```python
from build123d import *

# Parameters (mm, degrees)
BOSS_EXTRUDE1_DEPTH = 3.175
SKETCH2_R           = 4.7625
CUT_EXTRUDE1_DEPTH  = 7.35


with BuildPart() as part:
    # Sketch1 → Boss-Extrude1 (new body, symmetric)
    with BuildSketch(Plane(origin=(0, 0, 0), x_dir=(1, 0, 0), z_dir=(0, 1, 0))):
        Polygon((-58.039, -19.304), (-58.039, -58.039), (-19.304, -58.039), (-19.304, -38.1), (19.304, -38.1), (19.304, -58.039), (58.039, -58.039), (58.039, -19.304), (38.1, -19.304), (38.1, 19.304), (58.039, 19.304), (58.039, 58.039), (19.304, 58.039), (19.304, 38.1), (-19.304, 38.1), (-19.304, 58.039), (-58.039, 58.039), (-58.039, 19.304), (-38.1, 19.304), (-38.1, -19.304), align=None)
    extrude(amount=BOSS_EXTRUDE1_DEPTH, both=True)

    # Sketch2 → Cut-Extrude1 (cut, through all)
    with BuildSketch(Plane(origin=(0, 3.175, 0), x_dir=(1, 0, 0), z_dir=(0, 1, 0))):
        with Locations((-22.86, 22.86)):
            Circle(SKETCH2_R)
        with Locations((-22.86, -22.86)):
            Circle(SKETCH2_R)
        with Locations((22.86, -22.86)):
            Circle(SKETCH2_R)
        with Locations((22.86, 22.86)):
            Circle(SKETCH2_R)
    extrude(amount=-CUT_EXTRUDE1_DEPTH, mode=Mode.SUBTRACT)


solid = part.part
```
Could you check a few things on this model? Use its own coordinates, in mm. A direction names the side the tool comes from. Round coordinates to 2 decimals unless told otherwise and drop trailing zeros. Loops run counter-clockwise (first coordinate to the right, second up) from the corner with the lowest first, then second, coordinate; pieces in that order, holes last.
Q1. On a 3-axis mill with a long thin cutter (end or side, diameter ignored), from which of +Z, -Z, +X, -X, +Y, -Y can I reach the whole of each face in a straight line? I mean faces 4 (the flat face through (19.304, 0, 48)), 5 (the flat face through (-39, 0, 58.039)), 6 (the flat face through (-38.1, 0, 0)), 7 (the flat face through (38.1, 0, 0)), 8 (the flat face through (-19.304, 0, -48)). Say none if no direction works.
Q2. Thinking about a two-plate mould opening in Z: for faces 1 (the flat face through (-19.304, 0, 48)), 2 (the flat face through (0, 0, 38.1)), 3 (the flat face through (48, 0, 19.304)), which applies, pulls with the +Z half, pulls with the -Z half, needs draft (parallel to the pull), parting line crosses it, or undercut?
Q3. I want a section at C-C (x = -45). Write out the boundary of the cut face in (y, z) (3 decimals).
Q4. I want a section at B-B (y = -1.75). Write out the boundary of the cut face in (x, z) (1 decimal).
Q5. Please list where these lines run through material, in increasing order: L1, parallel to Z at x = -22.86, y = -1.5; L2, parallel to Z at x = -38.5, y = 1.25.
Q6. For P1, Ø1.9, axis at x = -4.5, y = 1, coming from the -Z side; P2, Ø1.9, axis at y = -0.5, z = -5, coming from the -X side; P3, Ø3, axis at y = 0.5, z = -8.5, coming from the +X side, each with a flat end and sliding along its axis, tell me the tip position at first contact or that it passes through.
Q7. I want a section at A-A (x = 22.86). Write out the boundary of the cut face in (y, z) (1 decimal).
Q8. I want a section at D-D (z = 46.5). Write out the boundary of the cut face in (x, y) (3 decimals).
Answer below:
1. face 4: +Z, +Y, -Y
1. face 5: +Z, +X, -X, +Y, -Y
1. face 6: -X, +Y, -Y
1. face 7: +X, +Y, -Y
1. face 8: -Z, +Y, -Y
2. face 1: needs draft
2. face 2: pulls with the +Z half
2. face 3: undercut
3. outline: (-3.175, -58.039) - (3.175, -58.039) - (3.175, -19.304) - (-3.175, -19.304) - close; (-3.175, 19.304) - (3.175, 19.304) - (3.175, 58.039) - (-3.175, 58.039) - close
4. outline: (-58, -58) - (-19.3, -58) - (-19.3, -38.1) - (19.3, -38.1) - (19.3, -58) - (58, -58) - (58, -19.3) - (38.1, -19.3) - (38.1, 19.3) - (58, 19.3) - (58, 58) - (19.3, 58) - (19.3, 38.1) - (-19.3, 38.1) - (-19.3, 58) - (-58, 58) - (-58, 19.3) - (-38.1, 19.3) - (-38.1, -19.3) - (-58, -19.3) - close; hole circle Ø9.5 at (-22.9, -22.9); hole circle Ø9.5 at (-22.9, 22.9); hole circle Ø9.5 at (22.9, -22.9); hole circle Ø9.5 at (22.9, 22.9)
5. L1: z = -58.04 to -27.62, -18.1 to 18.1, 27.62 to 58.04
5. L2: z = -58.04 to -19.3, 19.3 to 58.04
6. P1: stops at z = -38.1
6. P2: stops at x = -38.1
6. P3: stops at x = 38.1
7. outline: (-3.2, -58) - (3.2, -58) - (3.2, -27.6) - (-3.2, -27.6) - close; (-3.2, -18.1) - (3.2, -18.1) - (3.2, 18.1) - (-3.2, 18.1) - close; (-3.2, 27.6) - (3.2, 27.6) - (3.2, 58) - (-3.2, 58) - close
8. outline: (-58.039, -3.175) - (-19.304, -3.175) - (-19.304, 3.175) - (-58.039, 3.175) - close; (19.304, -3.175) - (58.039, -3.175) - (58.039, 3.175) - (19.304, 3.175) - close
